Solid Edge part; units mm, degrees
sketch "Sketch1" plane through (0, 0, 0) normal (0, 0, 1) x (1, 0, 0)
  circle A0 centre (0, 0) radius 8
  circle A1 centre (0, 0) radius 2
extrude "Protrusion1" add sketch "Sketch1" along normal blind 10
sketch "Sketch2" plane through (0, 0, 10) normal (0, 0, 1) x (1, 0, 0)
  circle A0 centre (0, 0) radius 5.15
extrude "VaciadoExtruido_1" cut sketch "Sketch2" against normal blind 8
sketch "Sketch3" plane through (0, 0, 10) normal (0, 0, 1) x (1, 0, 0)
  circle A0 centre (0, 0) radius 7
extrude "VaciadoExtruido_2" cut sketch "Sketch3" against normal blind 5 flip side to cut
chamfer "Chaflán_1" distance 1 angle 45 1 edges at (-2, 0, 0)
CAD build for the part. Positions are in the model's coordinates, mm. A direction names the side the tool comes from. Coordinates: 2 decimals unless noted, no trailing zeros. Order: outer loops, then holes, each group sorted by start corner. A loop starts at its lowest first (then second) coordinate and runs counter-clockwise, first axis right, second up. Notation, with made-up numbers: (16.25, 15.5) -> (46.25, 15.5) arc R20 cw to (46.25, 33.5) -> close; hole circle Ø3 at (21, 28). An arc over 180 degrees is marked (long way). Answer in a Markdown table with one row per item.
1) Band-saw the part on A-A (x = 0). List the corners of the cut face in (y, z), and give its area (3 significant figures).
Check values:
| item | result |
|---|---|
| outline | (-8, 0) -> (-3, 0) -> (-2, 1) -> (-2, 2) -> (-5.15, 2) -> (-5.15, 10) -> (-7, 10) -> (-7, 5) -> (-8, 5) -> close; (2, 1) -> (3, 0) -> (8, 0) -> (8, 5) -> (7, 5) -> (7, 10) -> (5.15, 10) -> (5.15, 2) -> (2, 2) -> close |
| area | 58.6 mm2 |
2) Band-saw the part on D-D (y = 3.25). List the corners of the cut face in (x, z) (3 decimals), and give its area (3 significant figures).
Check values:
| item | result |
|---|---|
| outline | (-7.31, 0) -> (7.31, 0) -> (7.31, 5) -> (6.2, 5) -> (6.2, 10) -> (3.995, 10) -> (3.995, 2) -> (-3.995, 2) -> (-3.995, 10) -> (-6.2, 10) -> (-6.2, 5) -> (-7.31, 5) -> close |
| area | 71.2 mm2 |
3) Band-saw the part on C-C (z = 7.5). List the corners of the cut face in (x, y), and give its area (3 significant figures).
Check values:
| item | result |
|---|---|
| outline | circle Ø14 at (0, 0); hole circle Ø10.3 at (0, 0) |
| area | 70.6 mm2 |
4) Mould opens along X. For faces 1 (the face through (-4, 4, 10)), 2 (the face through (-1.73, 7.81, 2.46)), 3 (the face through (-0.1, -2.2, 2)) say: pulls with the +X half, pulls with the -X half, needs draft (parallel to the pull), parting line crosses it, or undercut.
Check values:
| item | result |
|---|---|
| face 1 | needs draft |
| face 2 | parting line crosses it |
| face 3 | undercut |
5) Drill centre lines: line 1 (Y direction, x = 0, z = 8); line 2 (X direction, y = 0, z = 1.6). Where is each one in solid material? Low to high.
Check values:
| item | result |
|---|---|
| line 1 | -7 to -5.15, 5.15 to 7 |
| line 2 | -8 to -2, 2 to 8 |
6) Flat gauge pins, fed straight in: P1, Ø1.5, axis at x = -2.5, z = 3, coming from the -Y side; P2, Ø1, axis at x = -1.5, z = 4.5, coming from the +Y side; P3, Ø1.5, axis at x = 0.5, z = 7, coming from the -Y side. Where does each tip first touch, or does it go through?
Check values:
| item | result |
|---|---|
| P1 | y = -7.81 |
| P2 | y = 7.94 |
| P3 | y = -7 |
7) Which spindle directions (+Z, -Z, +X, -X, +Y, -Y) get a long thin tool onto all of the face, cutting with end or side? Do faces 4 (the face through (4.91, 1.55, 6.06)), 5 (the face through (3.4, 0.1, 0)). Say none if no direction does.
Check values:
| item | result |
|---|---|
| face 4 | +Z |
| face 5 | -Z, +X, -X, +Y, -Y |
